Source: CAD feature listing. Evaluate the final solid. Frame: model axes, mm. A direction names the side the tool comes from. Round coordinates to 2 decimals unless told otherwise and drop trailing zeros. Loops run counter-clockwise (first coordinate to the right, second up) from the corner with the lowest first, then second, coordinate; pieces in that order, holes last.
Item 1: Section query A-A on x = 1.1. Return loops of the section in (y, z).
Item 2: Access query for faces 1 (the flat face through (1, -30, 4)), 2 (the flat face through (1, 29, 7)), 3 (the flat face through (1, -31, -4)). Directions: +Z, -Z, +X, -X, +Y, -Y. A direction counts if a zero-diameter tool reaches every point of the face in a straight line with its end or side. Return the directions, or none.
Item 3: Ray query, L1, parallel to Y at x = 2.85, z = 6. Return the intervals inside material, ascending.
Item 4: First-contact query: P1, Ø1.5, axis at x = 2, z = 9, coming from the +Y side. Flat tip, straight axial feed; report the tip coordinate or a pass-through.
Item 5: Section query B-B on z = -5.25. Return loops of the section in (x, y), then the cut area to 3 significant figures.
```python
from build123d import *

# Parameters (mm, degrees)
F1_DEPTH = 3


with BuildPart() as f1:
    # F0 (on Right) → F1 (new body)
    with BuildSketch(Plane.YZ):
        Polygon((-32, 4), (-32, 0), (-32, -4), (-29, -4), (-29, -7), (0, -7), (29, -7), (29, -4), (32, -4), (32, 0), (32, 4), (29, 4), (29, 11), (0, 11), (-29, 11), (-29, 4), align=None)
    extrude(amount=F1_DEPTH)


solid = f1.part
```
Data:
1. outline: (-32, -4) - (-29, -4) - (-29, -7) - (29, -7) - (29, -4) - (32, -4) - (32, 4) - (29, 4) - (29, 11) - (-29, 11) - (-29, 4) - (-32, 4) - close
2. face 1: +Z, +X, -X, -Y
2. face 2: +Z, +X, -X, +Y
2. face 3: -Z, +X, -X, -Y
3. L1: y = -29 to 29
4. P1: stops at y = 29
5. outline: (0, -29) - (3, -29) - (3, 29) - (0, 29) - close
5. area: 174 mm2
